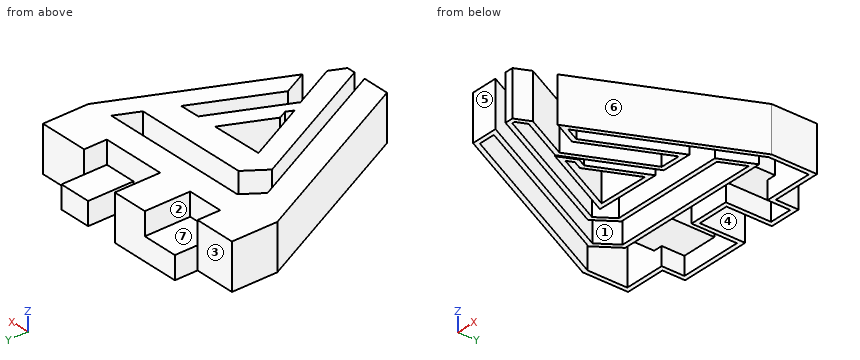
from build123d import *

# Parameters (mm, degrees)
SKETCH_2_W          = 199.99999999999972
SKETCH_2_H          = 40.0000000000029
EXTRUDE_1_DEPTH     = 40
EXTRUDE_5_DEPTH     = 20
CUT_EXTRUDE_1_DEPTH = 20
SHELL_1_T           = -4


with BuildPart() as part:
    # Sketch 2 → Extrude 1 (new body)
    # profile 1 of 2: a face of its own
    with BuildSketch(Plane.XY):
        Polygon((-292.83766907737163, -36.600636615400134), (-492.83766907737134, -36.600636615400134), (-411.04350764937084, -201.54780387004163), (-387.3021178796635, -201.54780387004163), (-459.64889501148184, -55.65235437147672), (-447.824430393232, -38.845349288689015), (-314.51618126146934, -38.84534928868898), (-323.84350707219164, -58.973746582631264), (-425.06859632409555, -58.973746582631264), (-438.13417767710234, -77.54484466606092), (-376.6434698856671, -201.54780387004163), (-369.27276463278196, -201.54780387004163), (-363.24825517120325, -188.54689424122049), (-383.08030790431167, -148.55331936912614), (-352.9457720883425, -83.52289998835491), (-335.1213284507255, -83.31131920781937), (-366.59780107826595, -151.23764228433387), (-355.9291354649939, -172.7522117911716), align=None)
        Polygon((-388.745435454288, -138.64702410749163), (-415.7109887551389, -84.26793942985627), (-370.4625020076991, -83.73082812704564), (-389.6473299690999, -125.13174485915943), (-385.9436191741513, -132.60069610569766), align=None, mode=Mode.SUBTRACT)
    # profile 2 of 2: a face of its own
    with BuildSketch(Plane.XY):
        with Locations((-392.8376690773715, -16.600636615398685)):
            Rectangle(SKETCH_2_W, SKETCH_2_H)
    extrude(amount=EXTRUDE_1_DEPTH)

    # Sketch 3 → Extrude 5 (add)
    with BuildSketch(Plane(origin=(0, 3.399363384602765, 0), x_dir=(1, 0, 0), z_dir=(0, 1, 0))):
        Polygon((-336.3917831998655, -20.00000000000003), (-336.3917831998655, -5.981e-14), (-364.61472613861844, -3.469e-14), (-364.61472613861844, -20.000000000000018), align=None)
        Polygon((-392.8376690773715, -3.469e-14), (-456.3917831998654, -3.469e-14), (-456.3917831998654, -20.00000000000002), (-424.61472613861844, -20.000000000000018), (-424.61472613861844, -40), (-392.8376690773715, -39.999999999999986), align=None)
    extrude(amount=EXTRUDE_5_DEPTH)

    # Sketch 3_6 → Cut-Extrude 1 (cut)
    with BuildSketch(Plane(origin=(0, 3.399363384602765, 0), x_dir=(1, 0, 0), z_dir=(0, 1, 0))):
        Polygon((-364.61472613861844, -20.000000000000018), (-364.61472613861844, -6.04e-14), (-392.8376690773715, -3.469e-14), (-392.8376690773715, -39.99999999999998), (-336.3917831998655, -39.99999999999998), (-336.3917831998655, -20.00000000000003), align=None)
        Polygon((-424.61472613861844, -20.00000000000001), (-456.39178319986536, -20.000000000000014), (-456.3917831998654, -40.00000000000006), (-424.61472613861844, -39.99999999999999), align=None)
    extrude(amount=-CUT_EXTRUDE_1_DEPTH, mode=Mode.SUBTRACT)

    # Shell 1
    shell_1_openings = [part.faces().sort_by_distance(p)[0] for p in [
        (-393.958302549, -65.824912477, 0),
    ]]
    offset(amount=SHELL_1_T, openings=shell_1_openings, kind=Kind.INTERSECTION)


solid = part.part
Work out the finished part from the listing and answer in its coordinate system (mm). Face numbers are marked on the shaded views. A direction names the side the tool comes from. Round coordinates to 2 decimals unless told otherwise and drop trailing zeros. Loops run counter-clockwise (first coordinate to the right, second up) from the corner with the lowest first, then second, coordinate; pieces in that order, holes last. Notation, with made-up numbers: (-31, -26) -> (9, -26) arc R13 cw to (9, -3) -> close; hole circle Ø2 at (-5, -24). An arc over 180 degrees is marked (long way). Use one line per item in the form item = value.
(1) Find section B-B on x = -348. Give the vertices of the cut face in (y, z), then the cut area to 3 significant figures.
Answer list:
outline = (-155.64, 0) -> (-146.13, 0) -> (-146.13, 36) -> (-120.62, 36) -> (-120.62, 0) -> (-111.1, 0) -> (-111.1, 40) -> (-155.64, 40) -> close; (-83.46, 0) -> (-79.46, 0) -> (-79.46, 36) -> (-62.97, 36) -> (-62.97, 0) -> (-58.97, 0) -> (-58.97, 40) -> (-83.46, 40) -> close; (-38.85, 0) -> (-34.85, 0) -> (-34.85, 36) -> (-20.6, 36) -> (-20.6, 16) -> (19.4, 16) -> (19.4, 0) -> (23.4, 0) -> (23.4, 20) -> (-16.6, 20) -> (-16.6, 40) -> (-38.85, 40) -> close
area = 1,790 mm2
(2) A tool of negligible diameter and unlimited length cuts with its end or side. For the marked faces 1, 2, 3 and 4, from which of +Z, -Z, +X, -X, +Y, -Y can it reach the whole face along a straight path? Write none if from no direction.
Answer list:
face_1 = +Z, -Z
face_2 = +Z, +Y
face_3 = +Z, -Z, -X, +Y
face_4 = +Z, -Z, +Y
(3) Find section C-C on y = -28. Give the vertices of the cut face in (x, z).
Answer list:
outline = (-492.84, 0) -> (-488.84, 0) -> (-488.84, 36) -> (-296.84, 36) -> (-296.84, 0) -> (-292.84, 0) -> (-292.84, 40) -> (-492.84, 40) -> close
(4) Straight lines are drawn through the part: line 1 (Y direction, x = -392.5, z = 36.5); line 2 (X direction, y = -53, z = 7); line 3 (X direction, y = -41, z = 10). For each, find the intervals that lie inside material, in ascending order.
Answer list:
line_1 = -201.55 to -191.07, -169.57 to -131.08, -83.99 to -58.97, -38.85 to -16.6
line_2 = -484.71 to -480.24, -462.67 to -457.78, -321.08 to -316.67, -304.85 to -300.44
line_3 = -490.66 to -486.19, -454.23 to -449.34, -315.51 to -311.11, -299.28 to -294.88
(5) Flat-ended cylindrical pins translate along their axes: P1, Ø1, axis at y = -165, z = 15, coming from the +X side; P2, Ø22, axis at x = -437.5, z = 28.5, coming from the +Y side; P3, Ø8, axis at y = -129, z = 30, coming from the +X side; P4, Ø17.5, axis at x = -350, z = 4, coming from the -Y side. Find the tip coordinate at first contact, or state that the pin passes through.
Answer list:
P1 = -352.11
P2 = 23.4
P3 = -333.8
P4 = -172.75
(6) For a pull along X with two mould halves and no side action, classify the marked faces 5, 6 and 7 as released by +X, released by -X, zero draft, split by the parting line, or undercut.
Answer list:
face_5 = zero draft
face_6 = released by +X
face_7 = undercut
(7) Find section A-A on y = -91. Give the number of separate pieces and of enclosed holes in the cut face, then the cut area to 3 significant figures.
Answer list:
separate_pieces = 4
enclosed_holes = 0
area = 1,600 mm2
